The drawing under review shows one solid part. Ordinate dimensions are in mm from its lowest x, y, z. A direction names the side the tool comes from. Coordinates: 2 decimals unless noted, no trailing zeros. Loops run counter-clockwise (first coordinate to the right, second up) from the corner with the lowest first, then second, coordinate; pieces in that order, holes last. Notation, with made-up numbers: M 7.25,30 L 57.25,30 A26 ccw 57.25,46 Z; hole C 27.25,68 d5. An arc over 180 degrees is marked long. Answer as a JSON object with one key per item and string values. Group by question number.
1. Insertion check: pin 1 (1.8 mm diameter, centred on x = 2, z = 23.5, fed in from -Y); pin 2 (4 mm diameter, centred on x = 19.5, z = 25, fed in from -Y); pin 3 (6.5 mm diameter, centred on y = 14.5, z = 16.5, fed in from -X); pin 4 (12 mm diameter, centred on x = 8, y = 6.5, fed in from -Z). Each pin has a flat end and moves straight along its axis. Give the tip position at first contact, or say it passes through.
2. Consider section C-C (x = 20.5). State the section outline as (y, z) points.
3. Consider section A-A (y = 11). State the section outline as (x, z) points, then the cut area to 3 significant figures.
4. Consider section D-D (z = 3). State the section outline as (x, y) points, then the cut area to 3 significant figures.
5. Consider section B-B (z = 16). State the section outline as (x, y) points, then the cut area to 3 significant figures.
6. Machinability: for the marked faces 1, 2, 3, 4 and 5, which of the approach directions +Z, -Z, +X, -X, +Y, -Y give a long, thin tool a straight path to every point of the face, cutting with its end or side? Answer none if there is none.
7. To check wall thickness, follow probe 1 along X at (y, z) = (3, 20); probe 2 along X at (y, z) = (6.5, 2); probe 3 along Y at (x, z) = (1.5, 21). State the ranges of each line that lie inside material, in increasing order.
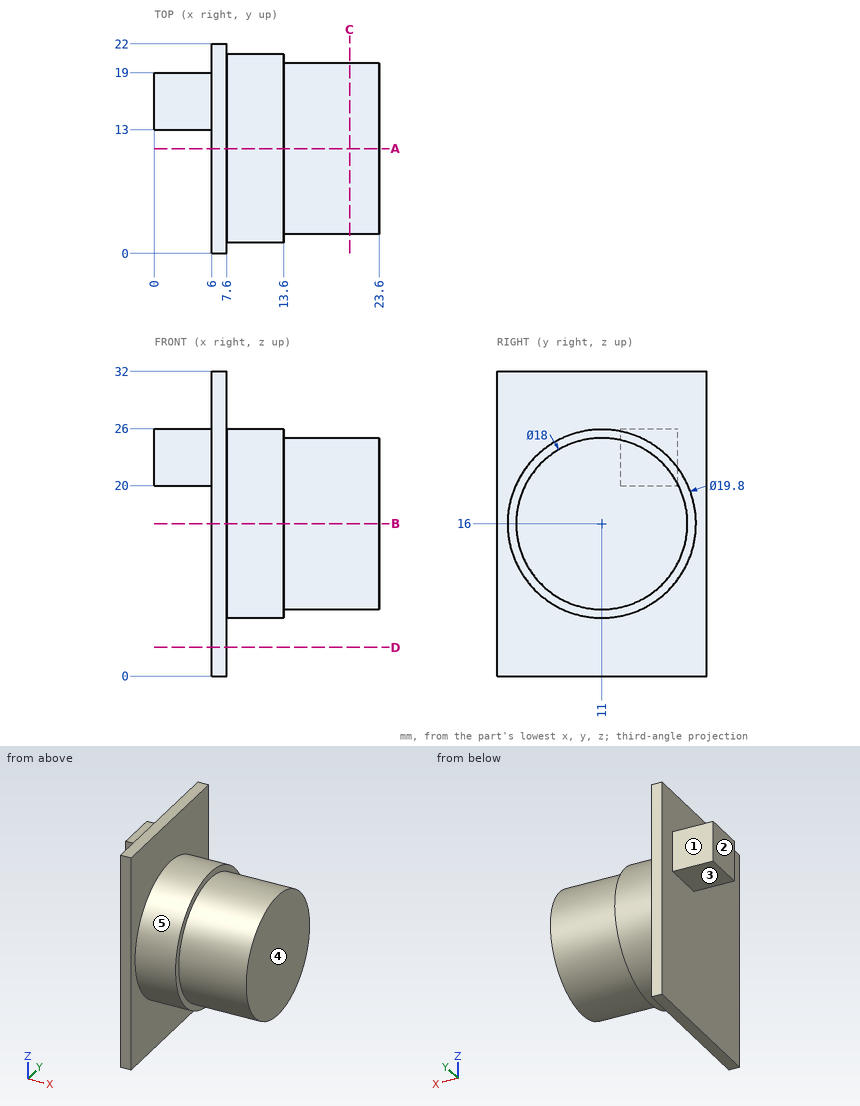
Findings below:
{
 "1": {"pin 1": "stops at y = 13", "pin 2": "stops at y = 5.34", "pin 3": "stops at x = 6", "pin 4": "stops at z = 0"},
 "2": {"outline": "C 11,16 d18"},
 "3": {"outline": "M 6,0 L 7.6,0 L 7.6,6.1 L 13.6,6.1 L 13.6,7 L 23.6,7 L 23.6,25 L 13.6,25 L 13.6,25.9 L 7.6,25.9 L 7.6,32 L 6,32 Z", "area": "350 mm^2"},
 "4": {"outline": "M 6,0 L 7.6,0 L 7.6,22 L 6,22 Z", "area": "35.2 mm^2"},
 "5": {"outline": "M 6,0 L 7.6,0 L 7.6,1.1 L 13.6,1.1 L 13.6,2 L 23.6,2 L 23.6,20 L 13.6,20 L 13.6,20.9 L 7.6,20.9 L 7.6,22 L 6,22 Z", "area": "334 mm^2"},
 "6": {"face 1": "+Z, -Z, -X, +Y", "face 2": "+Z, -Z, -X, +Y, -Y", "face 3": "-Z, -X, +Y, -Y", "face 4": "+Z, -Z, +X, +Y, -Y", "face 5": "+X"},
 "7": {"probe 1": "x = 6 to 23.6", "probe 2": "x = 6 to 7.6", "probe 3": "y = 13 to 19"}
}
